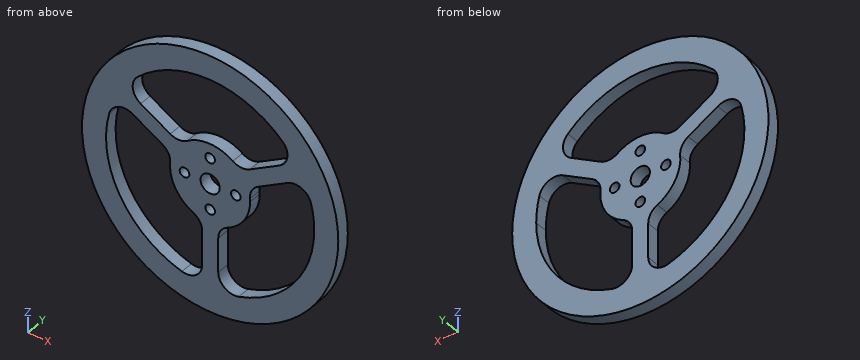
```python
from build123d import *

# Parameters (mm, degrees)
SKETCH_1_R          = 40
EXTRUDE_1_DEPTH     = 4
SKETCH_2_R          = 1.5
SKETCH_2_R_2        = 3
CUT_EXTRUDE_1_DEPTH = 5
CUT_EXTRUDE_2_DEPTH = 10
FILLET_1_R          = 5


with BuildPart() as part:
    # 草图1 → 凸台-拉伸1 (new body)
    with BuildSketch(Plane(origin=(0, 0, 0), x_dir=(1, 0, 0), z_dir=(0, 1, 0))):
        Circle(SKETCH_1_R)
    extrude(amount=EXTRUDE_1_DEPTH)

    # 草图2 → 切除-拉伸1 (cut, through all)
    with BuildSketch(Plane(origin=(0, 4, 0), x_dir=(1, 0, 0), z_dir=(0, 1, 0))):
        with Locations((8, 0)):
            Circle(SKETCH_2_R)
        with Locations((0, 8)):
            Circle(SKETCH_2_R)
        with Locations((-8, 0)):
            Circle(SKETCH_2_R)
        with Locations((0, -8)):
            Circle(SKETCH_2_R)
        Circle(SKETCH_2_R_2)
    extrude(amount=-CUT_EXTRUDE_1_DEPTH, mode=Mode.SUBTRACT)

    # 草图3 → 切除-拉伸2 (cut)
    with BuildSketch(Plane(origin=(0, 4, 0), x_dir=(1, 0, 0), z_dir=(0, 1, 0))):
        with BuildLine():
            Line((-29.324463582, -14.011632155), (-11.86555962, -3.931729252))
            ThreePointArc((-11.86555962, -3.931729252), (-10.811101802, 6.274557978), (-2.472197603, 12.253090998))
            Line((-2.472197603, 12.253090998), (-2.472197603, 32.405836496))
            ThreePointArc((-2.472197603, 32.405836496), (-28.131872753, 16.274143154), (-29.324463582, -14.011632155))
        make_face()
        with BuildLine():
            ThreePointArc((12.5, 0), (12.335818498, -2.019302353), (11.847586881, -3.985559571))
            Line((11.847586881, -3.985559571), (29.300376438, -14.06193232))
            ThreePointArc((29.300376438, -14.06193232), (31.69000027, -7.210678392), (32.5, 0))
            ThreePointArc((32.5, 0), (23.857950225, 22.069168789), (2.527802397, 32.401546492))
            Line((2.527802397, 32.401546492), (2.527802397, 12.241740687))
            ThreePointArc((2.527802397, 12.241740687), (9.691427396, 7.894696639), (12.5, 0))
        make_face()
        with BuildLine():
            Line((26.796661185, -18.389914337), (9.337757223, -8.310011435))
            ThreePointArc((9.337757223, -8.310011435), (-0.028375705, -12.499967793), (-9.375389278, -8.267531427))
            Line((-9.375389278, -8.267531427), (-26.828178835, -18.343904176))
            ThreePointArc((-26.828178835, -18.343904176), (-0.027885019, -32.499988037), (26.796661185, -18.389914337))
        make_face()
    extrude(amount=-CUT_EXTRUDE_2_DEPTH, mode=Mode.SUBTRACT)

    # 圆角1
    fillet_1_edges = [part.edges().sort_by_distance(p)[0] for p in [
        (11.847586881, 2, 3.985559571),
        (2.527802397, 2, -12.241740687),
        (2.527802397, 2, -32.401546492),
        (29.300376438, 2, 14.06193232),
        (-9.375389278, 2, 8.267531427),
        (9.337757223, 2, 8.310011435),
        (26.796661185, 2, 18.389914337),
        (-26.828178835, 2, 18.343904176),
        (-2.472197603, 2, -12.253090998),
        (-11.86555962, 2, 3.931729252),
        (-29.324463582, 2, 14.011632155),
        (-2.472197603, 2, -32.405836496),
    ]]
    fillet(fillet_1_edges, radius=FILLET_1_R)


solid = part.part
```
The listing builds one solid part. Answer for the finished solid, in the listing's coordinates (mm). Coordinates: 2 decimals unless noted, no trailing zeros. Write each loop counter-clockwise with the first axis right and the second up, starting at its lowest first coordinate (ties: lowest second). Pieces come first, ordered by that corner, then holes. Notation, with made-up numbers: (-32.75, 41.5) -> (-5.75, 41.5) arc R22 cw to (-5.75, 72.5) -> close; hole circle Ø10 at (66, -10). An arc over 180 degrees is marked (long way). Write each question's results on one line, items separated by ' | '. Start each with the question number.
1) Flat-ended cylindrical pins translate along their axes: pin 1 Ø2 at (y, z) = (1.5, -20) entering from +X; pin 2 Ø2 at (x, y) = (4.5, 3.5) entering from +Z; pin 3 Ø2 at (y, z) = (2, -24) entering from -X. Find the tip coordinate at first contact, or state that the pin passes through.
2) Straight lines are drawn through the part: probe 1 along Z at (x, y) = (0, 1.15); probe 2 along X at (y, z) = (1.85, 0); probe 3 along Z at (x, y) = (7, 0.5). For each, find the intervals that lie inside material, in ascending order.
3) A cutting plane is placed at C-C (z = -8). Determine the outline of the cut face in (x, y), then the cut area to 3 significant figures.
4) A cutting plane is placed at A-A (x = 0). Determine the outline of the cut face in (y, z).
5) A cutting plane is placed at B-B (z = 4). Determine the outline of the cut face in (x, y).
6) A cutting plane is placed at D-D (x = -27). Determine the outline of the cut face in (y, z).
Values follow:
1) pin 1: x = 35.2 | pin 2: z = 39.85 | pin 3: x = -32.73
2) probe 1: -40 to -9.5, -6.5 to -3, 3 to 6.5, 9.5 to 12.5, 32.5 to 40 | probe 2: -40 to -32.5, -12.5 to -9.5, -6.5 to -3, 3 to 6.5, 9.5 to 12.5, 32.5 to 40 | probe 3: -39.38 to -31.42, -10.36 to -1.12, 1.12 to 10.36, 31.74 to 39.38
3) outline: (-39.19, 0) -> (-31.5, 0) -> (-31.5, 4) -> (-39.19, 4) -> close; (-9.6, 0) -> (-1.5, 0) -> (-1.5, 4) -> (-9.6, 4) -> close; (1.5, 0) -> (9.6, 0) -> (9.6, 4) -> (1.5, 4) -> close; (31.5, 0) -> (39.19, 0) -> (39.19, 4) -> (31.5, 4) -> close | area: 126 mm²
4) outline: (0, -40) -> (4, -40) -> (4, -9.5) -> (0, -9.5) -> close; (0, -6.5) -> (4, -6.5) -> (4, -3) -> (0, -3) -> close; (0, 3) -> (4, 3) -> (4, 6.5) -> (0, 6.5) -> close; (0, 9.5) -> (4, 9.5) -> (4, 12.5) -> (0, 12.5) -> close; (0, 32.5) -> (4, 32.5) -> (4, 40) -> (0, 40) -> close
5) outline: (-39.8, 0) -> (-32.25, 0) -> (-32.25, 4) -> (-39.8, 4) -> close; (-13.19, 0) -> (13.14, 0) -> (13.14, 4) -> (-13.19, 4) -> close; (32.25, 0) -> (39.8, 0) -> (39.8, 4) -> (32.25, 4) -> close
6) outline: (0, -29.51) -> (4, -29.51) -> (4, -18.09) -> (0, -18.09) -> close; (0, 11.69) -> (4, 11.69) -> (4, 29.51) -> (0, 29.51) -> close
